Autodesk Inventor part; units mm, degrees
ref_plane "YZ Plane" through (0, 0, 0) normal (1, 0, 0) x (0, 1, 0)
ref_plane "XZ Plane" through (0, 0, 0) normal (0, 1, 0) x (-1, 0, 0)
ref_plane "XY Plane" through (0, 0, 0) normal (0, 0, 1) x (1, 0, 0)
sketch "スケッチ1" plane through (0, 0, 0) normal (0, 0, 1) x (1, 0, 0)
  circle A0 centre (0, 0) radius 5.2
  line L0 (25, -50) -> (-25, -50)
  line L1 (-25, -50) -> (-25, 50)
  line L2 (-25, 50) -> (25, 50)
  line L3 (25, 50) -> (25, -50)
  line L4 (25, -50) -> (-25, 50) construction
  line L5 (-25, -50) -> (25, 50) construction
  dimension "d0" = 10.4
  dimension "d1" = 50
  dimension "d2" = 100
extrude "押し出し1" add sketch "スケッチ1" along normal blind 3
sketch "スケッチ2" plane through (0, 0, 3) normal (0, 0, 1) x (1, 0, 0)
  circle A0 centre (17.3198, -9.9987) radius 1.25 construction
  circle A1 centre (-17.3213, -10.0013) radius 1.25 construction
  circle A2 centre (0.0015, -40) radius 1.25 construction
  line L0 (-17.3213, -10.0013) -> (-17.3213, -12.0013) construction
  line L1 (-18.9213, -10.0013) -> (-18.9213, -12.0013)
  line L2 (-15.7213, -12.0013) -> (-15.7213, -10.0013)
  arc A3 (-15.7213, -10.0013) -> (-18.9213, -10.0013) centre (-17.3213, -10.0013) ccw
  arc A4 (-18.9213, -12.0013) -> (-15.7213, -12.0013) centre (-17.3213, -12.0013) ccw
  line L3 (0.0015, -40) -> (0.0015, -42) construction
  line L4 (-1.5985, -40) -> (-1.5985, -42)
  line L5 (1.6015, -42) -> (1.6015, -40)
  arc A5 (1.6015, -40) -> (-1.5985, -40) centre (0.0015, -40) ccw
  arc A6 (-1.5985, -42) -> (1.6015, -42) centre (0.0015, -42) ccw
  line L6 (17.3198, -9.9987) -> (17.3198, -11.9987) construction
  line L7 (15.7198, -9.9987) -> (15.7198, -11.9987)
  line L8 (18.9198, -11.9987) -> (18.9198, -9.9987)
  arc A7 (18.9198, -9.9987) -> (15.7198, -9.9987) centre (17.3198, -9.9987) ccw
  arc A8 (15.7198, -11.9987) -> (18.9198, -11.9987) centre (17.3198, -11.9987) ccw
  circle A9 centre (0, 0) radius 5.2
  arc A10 (5.3111, 6.2476) -> (-5.3114, 6.2473) centre (0, 0) ccw
  line L9 (-12.7213, -12.0013) -> (-12.7213, -10.0013)
  arc A11 (-20.3008, -6.4967) -> (-21.9213, -10.0013) centre (-17.3213, -10.0013) ccw
  line L10 (-21.9213, -10.0013) -> (-21.9213, -12.0013)
  arc A12 (-21.9213, -12.0013) -> (-21.3048, -14.3016) centre (-17.3213, -12.0013) ccw
  line L11 (21.9198, -11.9987) -> (21.9198, -9.9987)
  arc A13 (21.9198, -9.9987) -> (20.2992, -6.494) centre (17.3198, -9.9987) ccw
  line L12 (12.7198, -9.9987) -> (12.7198, -11.9987)
  arc A14 (21.3037, -14.2984) -> (21.9198, -11.9987) centre (17.3198, -11.9987) ccw
  line L13 (4.6015, -40) -> (4.6015, -42)
  arc A15 (-3.9821, -44.3003) -> (3.9854, -44.2997) centre (0.0015, -42) ccw
  line L14 (-4.5985, -42) -> (-4.5985, -40)
  arc A16 (4.6015, -40) -> (-4.5985, -40) centre (0.0015, -40) ccw
  line L15 (-20.3008, -6.4967) -> (-5.3114, 6.2473)
  line L16 (5.3111, 6.2476) -> (20.2992, -6.494)
  line L17 (21.3037, -14.2984) -> (3.9854, -44.2997)
  line L18 (-3.9821, -44.3003) -> (-21.3048, -14.3016)
  point P0 (-17.3213, -11.0013)
  point P1 (0.0015, -41)
  point P2 (17.3198, -10.9987)
  dimension "d5" = 1.6
  dimension "d6" = 2
  dimension "d7" = 3
  dimension "d8" = 3
  dimension "d9" = 3
  dimension "d10" = 3
extrude "押し出し2" cut sketch "スケッチ2" against normal blind 3 keep common part
properties part number "POTplate" material "アルミニウム 2014-T4"
Could you check a few things on this model? Use its own coordinates, in mm. A direction names the side the tool comes from. Round coordinates to 2 decimals unless told otherwise and drop trailing zeros. Write each loop counter-clockwise with the first axis right and the second up, starting at its lowest first coordinate (ties: lowest second). Pieces come first, ordered by that corner, then holes. Notation, with made-up numbers: M 16,-21 L 58,-21 A11 ccw 58,-14 Z; hole C -31,73.5 d9. An arc over 180 degrees is marked long. Answer in a Markdown table with one row per item. Add a question column.
Q1. If we mould it in two halves opening along Y, with no side actions, what happens to faces 1 (the flat face through (-12.522, -29.511, 1.521)), 2 (the cylindrical face through (17.3, -13.6, 1.5)), 3 (the flat face through (-21.921, -11, 2))? For each: +Y half, -Y half, draft (parallel to the pull), parting line (faces both ways), or undercut.
Q2. Imagine slicing it at B-B (z = 1.9). Please give me the cut outline in (x, y), then the cut area to 3 significant figures.
Q3. Imagine slicing it at A-A (x = 0). Please give me the cut outline in (y, z), then the cut area to 3 significant figures.
Q4. Imagine slicing it at D-D (x = -17). Please give me the cut outline in (y, z), then the cut area to 3 significant figures.
Q5. Will these pins go through, and if not, where does the flat tip stop? pin 1 Ø10 at (x, y) = (17.5, -40) entering from -Z; pin 2 Ø1 at (y, z) = (-17, 1) entering from -X; pin 3 Ø1 at (x, z) = (9.5, 0.5) entering from +Y.
Q6. If I drill on line 1 (Y direction, x = 0, z = 0.9); line 2 (X direction, y = -9, z = 0.3); line 3 (Y direction, x = -2, z = 0.55), over which ranges is the centre line in solid material (lowest first)? Write a range as from..to.
Q7. Imagine slicing it at C-C (y = 0). Please give me the cut outline in (x, z), then the cut area to 3 significant figures.
Q8. On a 3-axis mill with a long thin cutter (end or side, diameter ignored), from which of +Z, -Z, +X, -X, +Y, -Y can I reach the whole of each face in a straight line? I mean faces 4 (the flat face through (12.766, -29.089, 1.521)), 5 (the flat face through (-15.721, -11, 2)). Say none if no direction works.
Values:
| question | item | result |
|---|---|---|
| 1 | face 1 | -Y half |
| 1 | face 2 | undercut |
| 1 | face 3 | draft |
| 2 | outline | M -21.92,-12 A4.6 ccw -21.3,-14.3 L -3.98,-44.3 A4.6 ccw 3.99,-44.3 L 21.3,-14.3 A4.6 ccw 21.92,-12 L 21.92,-10 A4.6 ccw 20.3,-6.49 L 5.31,6.25 A8.2 ccw -5.31,6.25 L -20.3,-6.5 A4.6 ccw -21.92,-10 Z; hole M -18.92,-12 A1.6 ccw -15.72,-12 L -15.72,-10 A1.6 ccw -18.92,-10 Z; hole C 0,0 d10.4; hole M -1.6,-42 A1.6 ccw 1.6,-42 L 1.6,-40 A1.6 ccw -1.6,-40 Z; hole M 15.72,-12 A1.6 ccw 18.92,-12 L 18.92,-10 A1.6 ccw 15.72,-10 Z |
| 2 | area | 1,320 mm^2 |
| 3 | outline | M -46.6,0 L -43.6,0 L -43.6,3 L -46.6,3 Z; M -38.4,0 L -5.2,0 L -5.2,3 L -38.4,3 Z; M 5.2,0 L 8.2,0 L 8.2,3 L 5.2,3 Z |
| 3 | area | 118 mm^2 |
| 4 | outline | M -21.76,0 L -13.57,0 L -13.57,3 L -21.76,3 Z; M -8.43,0 L -3.69,0 L -3.69,3 L -8.43,3 Z |
| 4 | area | 38.8 mm^2 |
| 5 | pin 1 | through |
| 5 | pin 2 | x = -20.04 |
| 5 | pin 3 | y = 3.11 |
| 6 | line 1 | -46.6..-43.6, -38.4..-5.2, 5.2..8.2 |
| 6 | line 2 | -21.81..-18.57, -16.07..16.07, 18.57..21.81 |
| 6 | line 3 | -46.14..-4.8, 4.8..7.95 |
| 7 | outline | M -12.66,0 L -5.2,0 L -5.2,3 L -12.66,3 Z; M 5.2,0 L 12.66,0 L 12.66,3 L 5.2,3 Z |
| 7 | area | 44.8 mm^2 |
| 8 | face 4 | +Z, -Z, +X, -Y |
| 8 | face 5 | +Z, -Z |
